Design review of the part shown in the three views and the two pictorial views. Dimensions are in mm from the part's minimum x, y and z. Round coordinates to 2 decimals unless told otherwise and drop trailing zeros. Order: outer loops, then holes, each group sorted by start corner. A loop starts at its lowest first (then second) coordinate and runs counter-clockwise, first axis right, second up.
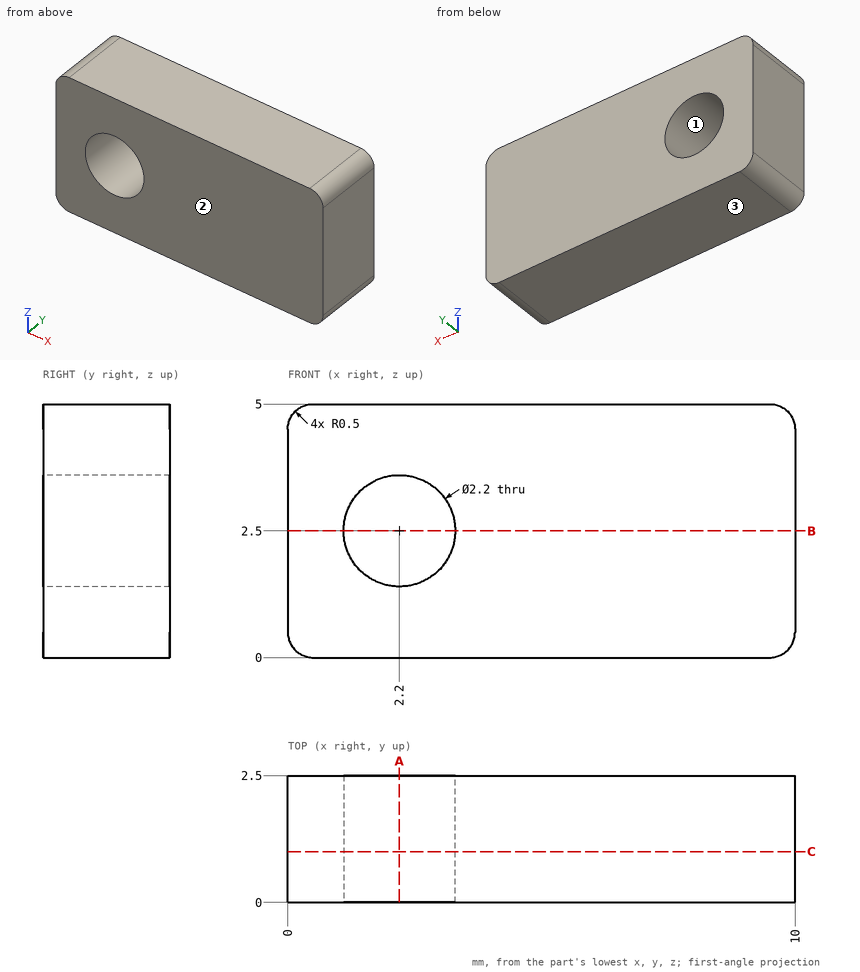
(1) Add section A-A on x = 2.2. Give the boundary of the cut face in (y, z), plus the area to 3 significant figures.
(2) Clearance check with a flat-ended pin moving along its axis: P1, Ø1.5, axis at x = 5, y = 1.5, coming from the -Z side. State where the tip first meets the part, or that it passes through.
(3) Add section B-B on z = 2.5. Give the boundary of the cut face in (x, y).
(4) Draft analysis for pull direction Z (two halves, no side actions). For the marked faces 1, 2 and 3, state which applies: pulls with the +Z half, pulls with the -Z half, needs draft (parallel to the pull), parting line crosses it, or undercut.
(5) Add section C-C on y = 1. Give the boundary of the cut face in (x, z).
(6) Wall thickness on L1, parallel to X at y = 0.55, z = 2.5; L2, parallel to Z at x = 2.2, y = 1.3; L3, parallel to X at y = 1.45, z = 3.4: over which ranges is each line inside the solid? List them lowest first.
Here are the results:
1. outline: (0, 0) - (2.5, 0) - (2.5, 1.4) - (0, 1.4) - close; (0, 3.6) - (2.5, 3.6) - (2.5, 5) - (0, 5) - close
1. area: 7.00 mm2
2. P1: stops at z = 0
3. outline: (0, 0) - (1.1, 0) - (1.1, 2.5) - (0, 2.5) - close; (3.3, 0) - (10, 0) - (10, 2.5) - (3.3, 2.5) - close
4. face 1: undercut
4. face 2: needs draft
4. face 3: pulls with the -Z half
5. outline: (0, 0.5) arc R0.5 ccw to (0.5, 0) - (9.5, 0) arc R0.5 ccw to (10, 0.5) - (10, 4.5) arc R0.5 ccw to (9.5, 5) - (0.5, 5) arc R0.5 ccw to (0, 4.5) - close; hole circle Ø2.2 at (2.2, 2.5)
6. L1: x = 0 to 1.1, 3.3 to 10
6. L2: z = 0 to 1.4, 3.6 to 5
6. L3: x = 0 to 1.57, 2.83 to 10
